Could you check a few things on this model? Use its own coordinates, in mm. A direction names the side the tool comes from. Give positions to 0.01 mm unless a question says otherwise; leave off trailing zeros. Loops run counter-clockwise (first coordinate to the right, second up) from the corner with the lowest first, then second, coordinate; pieces in that order, holes last. Notation, with made-up numbers: (24.25, -40) - (48.25, -40) arc R9 cw to (48.25, -28) - close; hole circle Ø8 at (53.25, 83.25). An arc over 180 degrees is marked (long way). Write each question's results on one line, items separated by ' | '. Start each with the question number.
1) I want a section at D-D, the plane y = 53. Write out the boundary of the cut face in (x, z).
2) If I drill on probe 1 along Y at (x, z) = (0, 0.05); probe 2 along X at (y, z) = (24, 0.7); probe 3 along Y at (x, z) = (2.5, 1.1), over which ranges is the centre line in solid material (lowest first)? Write a range as [from, to].
3) On a 3-axis mill with a long thin cutter (end or side, diameter ignored), from which of +Z, -Z, +X, -X, +Y, -Y can I reach the whole of each face in a straight line? I mean faces 5 (the face through (10, 26, 1)), 6 (the face through (0, 37, 2.5)), 7 (the face through (-10, 26, 1)). Say none if no direction works.
4) I want a section at C-C, the plane z = 2. Write out the boundary of the cut face in (x, y).
5) I'm going to push flat-ended pins straight in: pin 1 (2 mm diameter, centred on x = 12, y = 13, fed in from -Z); pin 2 (1 mm diameter, centred on x = -3.5, y = 51, fed in from -Z); pin 3 (0.8 mm diameter, centred on y = 25, z = 1, fed in from -X). Where does each tip first touch, or does it pass through?
6) If we mould it in two halves opening along Y, with no side actions, what happens to faces 1 (the face through (12.465, 61.86, 1.232)), 2 (the face through (0, 51, 0.6)), 3 (the face through (0, 62, 0)), 4 (the face through (0, 72, 1))? For each: +Y half, -Y half, draft (parallel to the pull), parting line (faces both ways), or undercut.
from build123d import *

# Parameters (mm, degrees)
DODANIE_WYCI_GNI_CIE1_DEPTH = 2.5
SZKIC2_W                    = 20
SZKIC2_H                    = 2
WYTNIJ_WYCI_GNI_CIE1_DEPTH  = 0.6
SZKIC3_R                    = 2.15
WYTNIJ_WYCI_GNI_CIE2_DEPTH  = 74.588382235
SFAZOWANIE1_SIZE2           = 2.5
SFAZOWANIE1_SIZE            = 2.7


with BuildPart() as part:
    # Szkic1 → Dodanie-wyciągnięcie1 (new body)
    with BuildSketch(Plane.XY):
        Polygon((-10, 0), (10, 0), (10, 50), (10, 52), (15, 72), (-15, 72), (-10, 52), (-10, 50), align=None)
    extrude(amount=DODANIE_WYCI_GNI_CIE1_DEPTH)

    # Szkic2 → Wytnij-wyciągnięcie1 (cut)
    with BuildSketch(Plane.XY):
        with Locations((0, 51)):
            Rectangle(SZKIC2_W, SZKIC2_H)
    extrude(amount=WYTNIJ_WYCI_GNI_CIE1_DEPTH, mode=Mode.SUBTRACT)

    # Szkic3 → Wytnij-wyciągnięcie2 (cut, through all)
    with BuildSketch(Plane.XY.offset(2.5)):
        with Locations((0, 10)):
            Circle(SZKIC3_R)
    extrude(amount=-WYTNIJ_WYCI_GNI_CIE2_DEPTH, mode=Mode.SUBTRACT)

    # Sfazowanie1
    sfazowanie1_edges = [part.edges().sort_by_distance(p)[0] for p in [
        (-2.15, 10, 2.5),
    ]]
    sfazowanie1_side = [part.faces().sort_by_distance(p)[0] for p in [
        (-2.2, 10, 2.5),
    ]]
    chamfer(sfazowanie1_edges, length=SFAZOWANIE1_SIZE - 0.0001, length2=SFAZOWANIE1_SIZE2 - 0.0001, reference=sfazowanie1_side[0])  # a hair under: the kernel refuses the full size


solid = part.part
Answers:
1) outline: (-10.25, 0) - (10.25, 0) - (10.25, 2.5) - (-10.25, 2.5) - close
2) probe 1: y = [0, 7.8], [12.2, 50], [52, 72] | probe 2: x = [-10, 10] | probe 3: y = [0, 7.79], [12.21, 72]
3) face 5: +Z, -Z, +X, -Y | face 6: +Z, +X, -X, +Y, -Y | face 7: +Z, -Z, -X, -Y
4) outline: (-15, 72) - (-10, 52) - (-10, 0) - (10, 0) - (10, 52) - (15, 72) - close; hole circle Ø8.62 at (0, 10)
5) pin 1: passes through | pin 2: stops at z = 0.6 | pin 3: stops at x = -10
6) face 1: -Y half | face 2: undercut | face 3: draft | face 4: +Y half
